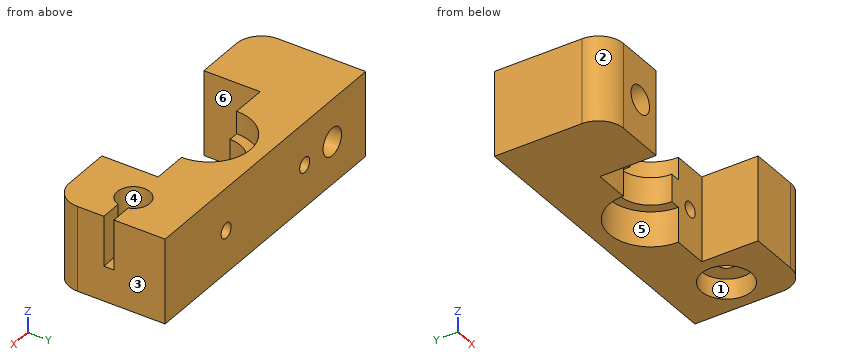
```python
from build123d import *

# Parameters (mm, degrees)
F1_DEPTH  = 8.5
F2_R      = 2.75
F3_DEPTH  = 22.501
F4_R      = 1.75
F5_DEPTH  = 17.001
F6_R      = 5
F7_DEPTH  = 4
F8_R      = 1.5
F9_DEPTH  = 11.251
F10_R     = 5
F12_DEPTH = 10
F15_DEPTH = 2.75


with BuildPart() as f1:
    # F0 (on Top) → F1 (new body, symmetric)
    with BuildSketch(Plane.XY):
        with BuildLine():
            ThreePointArc((-8.25, 0), (0, 8.25), (8.25, 0))
            Line((8.25, 0), (15.25, 0))
            Line((15.25, 0), (15.25, -11.25))
            Line((15.25, -11.25), (30, -11.25))
            Line((30, -11.25), (30, 11.25))
            Line((30, 11.25), (0, 11.25))
            Line((0, 11.25), (-30, 11.25))
            Line((-30, 11.25), (-30, 0))
            Line((-30, 0), (-30, -11.25))
            Line((-30, -11.25), (-15.25, -11.25))
            Line((-15.25, -11.25), (-15.25, 0))
            Line((-15.25, 0), (-8.25, 0))
        make_face()
    extrude(amount=F1_DEPTH, both=True)

    # F2 (on face) → F3 (cut, through all)
    with BuildSketch(Plane.XZ.offset(11.25)):
        with Locations((-20, 0)):
            Circle(F2_R)
    extrude(amount=-F3_DEPTH, mode=Mode.SUBTRACT)

    # F4 (on face) → F5 (cut, through all)
    with BuildSketch(Plane.XY.offset(8.5)):
        with Locations((22.625, 0)):
            Circle(F4_R)
    extrude(amount=-F5_DEPTH, mode=Mode.SUBTRACT)

    # F6 (on face) → F7 (cut)
    with BuildSketch(Plane(origin=(0, 0, -8.5), x_dir=(1, 0, 0), z_dir=(0, 0, -1))):
        with Locations((22.625, 0)):
            Circle(F6_R)
    extrude(amount=-F7_DEPTH, mode=Mode.SUBTRACT)

    # F8 (on face) → F9 (cut, through all)
    with BuildSketch(Plane.XZ):
        with Locations((-11.75, 0)):
            Circle(F8_R)
        with Locations((11.75, 0)):
            Circle(F8_R)
    extrude(amount=-F9_DEPTH, mode=Mode.SUBTRACT)

    # F10
    f10_edges = [f1.edges().sort_by_distance(p)[0] for p in [
        (-30, -11.25, 0),
        (30, -11.25, 0),
    ]]
    fillet(f10_edges, radius=F10_R)

    # F11 (on face) → F12 (cut)
    with BuildSketch(Plane.XY.offset(8.5)):
        with BuildLine():
            Line((30, 1), (25.7173292192, 1))
            ThreePointArc((25.7173292192, 1), (19.375, 0), (25.7173292192, -1))
            Line((25.7173292192, -1), (30, -1))
            Line((30, -1), (30, 0))
            Line((30, 0), (30, 1))
        make_face()
    extrude(amount=-F12_DEPTH, mode=Mode.SUBTRACT)

    # F14 (on offset) → F15 (join, symmetric)
    with BuildSketch(Plane.XY.offset(1.25)):
        with BuildLine():
            Line((6.25, 0), (9, 0))
            ThreePointArc((9, 0), (0, 9), (-9, 0))
            Line((-9, 0), (-6.25, 0))
            ThreePointArc((-6.25, 0), (0, 6.25), (6.25, 0))
        make_face()
    extrude(amount=F15_DEPTH, both=True)


solid = f1.part
```
The listing builds one solid part. Answer for the finished solid, in the listing's coordinates (mm). Face numbers are marked on the shaded views. A direction names the side the tool comes from. Round coordinates to 2 decimals unless told otherwise and drop trailing zeros. Order: outer loops, then holes, each group sorted by start corner. A loop starts at its lowest first (then second) coordinate and runs counter-clockwise, first axis right, second up. Notation, with made-up numbers: (-26.75, 22.25) - (-6.75, 22.25) arc R33 ccw to (-6.75, 52.25) - close; hole circle Ø8 at (27.5, -13). An arc over 180 degrees is marked (long way). Put each result on its own line as item: value. Start each with the question number.
(1) For the marked faces 4, 5 and 6, determine the directions among +Z, -Z, +X, -X, +Y, -Y from which every point of the face is accessible in a straight line to the end or side of a thin tool.
(2) Find section D-D (z = 7.25). Give the vertices of the cut face in (x, y) (3 decimals), plus the area to 3 significant figures.
(3) Determine the mould class of the marked faces 1, 2 and 3 for opening direction X: released by +X, released by -X, zero draft, split by the parting line, or undercut.
(4) Find section A-A (x = -11.75). Give the vertices of the cut face in (y, z), plus the area to 4 significant figures.
(5) Straight lines are drawn through the part: probe 1 along Z at (x, y) = (-20, -2.25); probe 2 along X at (y, z) = (-3, -4); probe 3 along X at (y, z) = (1.25, 6) (3 decimals). For each, find the intervals that lie inside material, in ascending order. Write a range as from..to.
(6) Given P1, Ø2.5, axis at x = 11, z = -1, coming from the -Y side; P2, Ø1.8, axis at x = 11.75, z = 0, coming from the -Y side; P3, Ø8.5, axis at x = 22.625, y = 0, coming from the -Z side; P4, Ø4, axis at y = -8.5, z = -4, coming from the +X side, each flat-ended and moving along its own axis, determine where each tip first touches the part or whether it passes through.
(7) Find section C-C (z = -5.75). Give the vertices of the cut face in (x, y) (3 decimals).
(8) Find section B-B (y = 9.25). Give the vertices of the cut face in (x, z).
Reply:
1. face 4: +Z
1. face 5: -Z, -Y
1. face 6: +Z, -Z, -Y
2. outline: (-30, -6.25) arc R5 ccw to (-25, -11.25) - (-15.25, -11.25) - (-15.25, 0) - (-8.25, 0) arc R8.25 cw to (8.25, 0) - (15.25, 0) - (15.25, -11.25) - (25, -11.25) arc R5 ccw to (30, -6.25) - (30, -1) - (25.717, -1) arc R3.25 cw (long way) to (25.717, 1) - (30, 1) - (30, 11.25) - (-30, 11.25) - close
2. area: 848 mm^2
3. face 1: undercut
3. face 2: released by -X
3. face 3: released by +X
4. outline: (0, -8.5) - (11.25, -8.5) - (11.25, -1.5) - (0, -1.5) - close; (0, 1.5) - (11.25, 1.5) - (11.25, 8.5) - (0, 8.5) - close
4. area: 157.5 mm^2
5. probe 1: -8.5..-2.75, 2.75..8.5
5. probe 2: -30..-15.25, 15.25..30
5. probe 3: -30..-8.155, 8.155..19.625, 25.625..30
6. P1: y = 0
6. P2: through
6. P3: z = -4.5
6. P4: x = 29.99
7. outline: (-30, -6.25) arc R5 ccw to (-25, -11.25) - (-15.25, -11.25) - (-15.25, 0) - (-8.25, 0) arc R8.25 cw to (8.25, 0) - (15.25, 0) - (15.25, -11.25) - (25, -11.25) arc R5 ccw to (30, -6.25) - (30, 11.25) - (-30, 11.25) - close; hole circle Ø10 at (22.625, 0)
8. outline: (-30, -8.5) - (30, -8.5) - (30, 8.5) - (-30, 8.5) - close; hole circle Ø5.5 at (-20, 0); hole circle Ø3 at (-11.75, 0); hole circle Ø3 at (11.75, 0)
